The figure shows three views and two pictorial views of one solid part (mm, origin at its lowest corner). Answer the questions. A direction names the side the tool comes from. Round coordinates to 2 decimals unless told otherwise and drop trailing zeros. Order: outer loops, then holes, each group sorted by start corner. A loop starts at its lowest first (then second) coordinate and runs counter-clockwise, first axis right, second up. Notation, with made-up numbers: (-23, -19.75) - (9, -19.75) arc R21 ccw to (9, 15.25) - close; hole circle Ø1 at (86.25, -36.5). An arc over 180 degrees is marked (long way). Use CSV: the item, a comma, the result in double quotes.
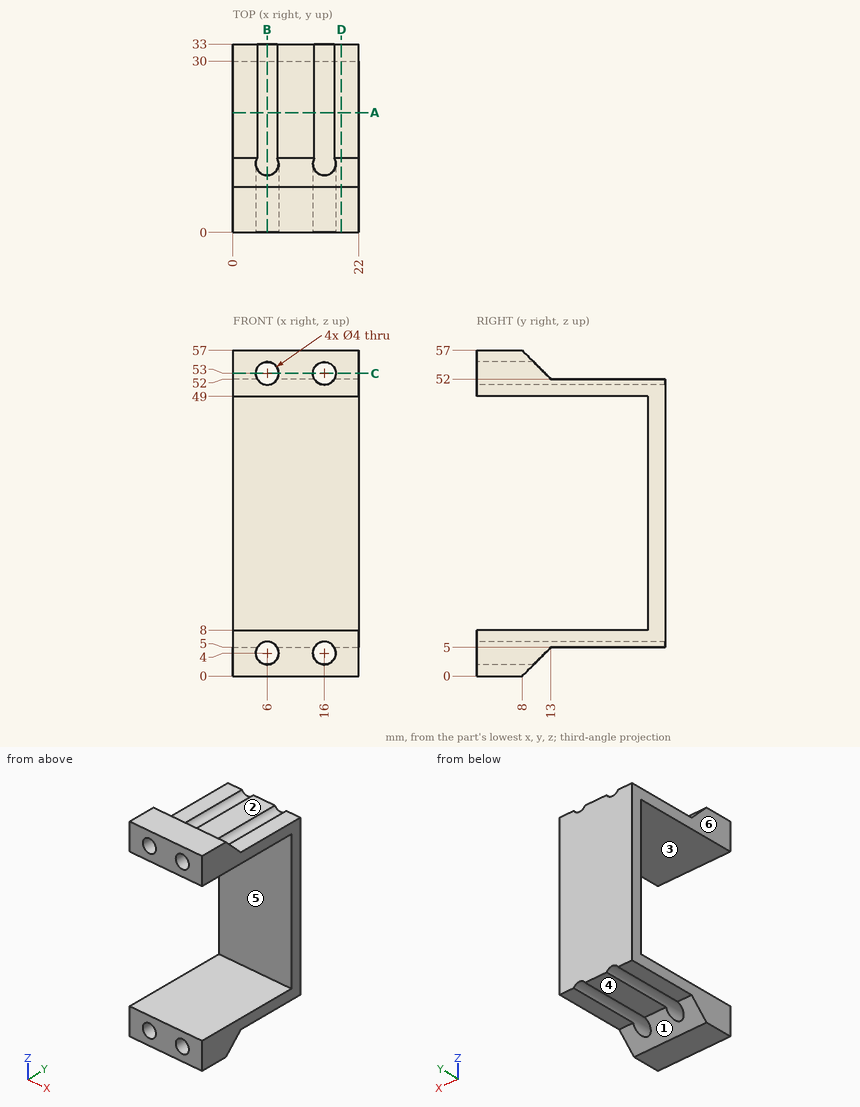
(1) Find the intervals of material crossed by L1, parallel to X at y = 4.5, z = 3; L2, parallel to X at y = 7, z = 53; L3, parallel to Z at x = 16, y = 26.5, in increasing order. Write a range as from..to.
Findings below:
L1,"x = 0..4.27, 7.73..14.27, 17.73..22"
L2,"x = 0..4, 8..14, 18..22"
L3,"z = 6..8, 49..51"
(2) Each of these flat-tipped pins is pushed along its axis until it touches: pin 1 (3.5 mm diameter, centred on x = 1.5, y = 26, fed in from +Z); pin 2 (2 mm diameter, centred on x = 12, y = 24, fed in from -Z); pin 3 (1.5 mm diameter, centred on x = 4, z = 23, fed in from -Y); pin 4 (10 mm diameter, centred on y = 21, z = 9.5, fed in from -X). Where does it stop, or does it pass through?
Findings below:
pin 1,"stops at z = 52"
pin 2,"stops at z = 5"
pin 3,"stops at y = 30"
pin 4,"stops at x = 0"
(3) Find section D-D (x = 19). Determine the outline of the cut face in (y, z), and give its area (3 significant figures).
Findings below:
outline,"(0, 0) - (8, 0) - (13, 5) - (33, 5) - (33, 52) - (13, 52) - (8, 57) - (0, 57) - (0, 49) - (30, 49) - (30, 8) - (0, 8) - close"
area,"426 mm²"
(4) For the marked faces 1, 2 and 3, determine the directions among +Z, -Z, +X, -X, +Y, -Y from which every point of the face is accessible in a straight line to the end or side of a thin tool.
Findings below:
face 1,"-Z, +X, -X, +Y"
face 2,"+Z, +X, -X, +Y"
face 3,"+X, -X, -Y"
(5) Find section B-B (x = 6). Determine the outline of the cut face in (y, z), and give its area (3 significant figures).
Findings below:
outline,"(0, 0) - (8, 0) - (10, 2) - (0, 2) - close; (0, 6) - (33, 6) - (33, 51) - (0, 51) - (0, 49) - (30, 49) - (30, 8) - (0, 8) - close; (0, 55) - (10, 55) - (8, 57) - (0, 57) - close"
area,"291 mm²"
(6) Find section A-A (y = 21). Determine the outline of the cut face in (x, z), and give its area (3 significant figures).
Findings below:
outline,"(0, 5) - (4.27, 5) arc R2 cw to (7.73, 5) - (14.27, 5) arc R2 cw to (17.73, 5) - (22, 5) - (22, 8) - (0, 8) - close; (0, 49) - (22, 49) - (22, 52) - (17.73, 52) arc R2 cw to (14.27, 52) - (7.73, 52) arc R2 cw to (4.27, 52) - (0, 52) - close"
area,"122 mm²"
(7) Find section C-C (z = 53). Determine the outline of the cut face in (x, y), and give its area (3 significant figures).
Findings below:
outline,"(0, 0) - (4, 0) - (4, 12) - (0, 12) - close; (8, 0) - (14, 0) - (14, 12) - (8, 12) - close; (18, 0) - (22, 0) - (22, 12) - (18, 12) - close"
area,"168 mm²"
(8) The mould has two halves that part along Z. Classify the marked faces 4, 5 and 6: released by +Z, released by -Z, zero draft, split by the parting line, or undercut.
Findings below:
face 4,"released by -Z"
face 5,"undercut"
face 6,"zero draft"
